Design review of the part built by this model. Coordinates are the model's own, in mm. Face numbers are marked on the shaded views. A direction names the side the tool comes from. Coordinates: 2 decimals unless noted, no trailing zeros. Loops run counter-clockwise (first coordinate to the right, second up) from the corner with the lowest first, then second, coordinate; pieces in that order, holes last. Notation, with made-up numbers: (36, 44) -> (75, 44) arc R11 ccw to (75, 60) -> close; hole circle Ø8 at (-13, -11). An arc over 180 degrees is marked (long way). One line per item, written item: value. Start each with the question number.
1. Add section B-B on z = -12. Write out the cut boundary in (x, y), plus the area to 3 significant figures.
2. Draft analysis for pull direction Z (two halves, no side actions). For the marked faces 4, 5 and 6, state which applies: pulls with the +Z half, pulls with the -Z half, needs draft (parallel to the pull), parting line crosses it, or undercut.
3. Machinability: for the marked faces 1, 2 and 3, which of the approach directions +Z, -Z, +X, -X, +Y, -Y give a long, thin tool a straight path to every point of the face, cutting with its end or side? Answer none if there is none.
4. For probe 1 along X at (y, z) = (11.5, 12); probe 2 along X at (y, z) = (12.75, -6.5); probe 3 along Z at (x, y) = (-4.5, 12), list the stretches that pass through material, from the lowest coordinate up.
5. Insertion check: pin 1 (2 mm diameter, centred on x = 14.5, y = 18.5, fed in from -Z); pin 2 (8 mm diameter, centred on x = 7, z = -13, fed in from +Y); pin 3 (3.5 mm diameter, centred on x = 13.5, z = -9.5, fed in from +Y). Each pin has a flat end and moves straight along its axis. Give the tip position at first contact, or say it passes through.
6. Add section A-A on y = 16. Write out the cut boundary in (x, z).
7. Add section C-C on y = 5.5. Write out the cut boundary in (x, z), plus the area to 3 significant figures.
8. Add section D-D on z = 21. Write out the cut boundary in (x, y).
Autodesk Inventor part; units mm, degrees
ref_plane "YZ Plane" through (0, 0, 0) normal (1, 0, 0) x (0, 1, 0)
ref_plane "XZ Plane" through (0, 0, 0) normal (0, 1, 0) x (-1, 0, 0)
ref_plane "XY Plane" through (0, 0, 0) normal (0, 0, 1) x (1, 0, 0)
sketch "Sketch1" plane through (0, 0, 0) normal (0, 0, 1) x (1, 0, 0)
  line L0 (16.85, 0) -> (-16.85, 0)
  line L1 (-16.85, 0) -> (-16.85, 20)
  line L2 (-16.85, 20) -> (-1.85, 20)
  line L3 (-1.85, 20) -> (-1.85, 7)
  line L4 (-1.85, 7) -> (1.85, 7)
  line L5 (1.85, 7) -> (1.85, 20)
  line L6 (1.85, 20) -> (16.85, 20)
  line L7 (16.85, 20) -> (16.85, 0)
  line L8 (-23.59, 0) -> (23.59, 0)
  line L9 (0, -4) -> (0, 24)
  point P0 (0, 0)
  point P1 (0, 7)
  point P2 (0, 0)
  dimension "d0" = 33.7
  dimension "d1" = 3.7
  dimension "d2" = 13
  dimension "d3" = 20
extrude "Extrusion1" add sketch "Sketch1" along normal mid plane 60
sketch "Sketch2" plane through (-16.85, 20, 30) normal (0, 1, 0) x (1, 0, 0)
  line L0 (0, 60) -> (0, 0)
  line L1 (15, 0) -> (0, 0)
  line L2 (15, 60) -> (15, 0)
  line L3 (0, 60) -> (15, 60)
  line L4 (18.7, 60) -> (18.7, 0)
  line L5 (33.7, 0) -> (18.7, 0)
  line L6 (33.7, 60) -> (33.7, 0)
  line L7 (18.7, 60) -> (33.7, 60)
  line L8 (25.85, 42) -> (7.85, 42) construction
  line L9 (7.85, 42) -> (7.85, 18) construction
  line L10 (7.85, 18) -> (25.85, 18) construction
  line L11 (25.85, 18) -> (25.85, 42) construction
  line L12 (25.85, 42) -> (7.85, 18) construction
  line L13 (7.85, 42) -> (25.85, 18) construction
  point P0 (16.85, 30)
  dimension "d6" = 18
  dimension "d7" = 24
hole "Hole1" at (-9, 20, 12) at (-9, 20, -12) at (9, 20, 12) at (9, 20, -12) direction (0, -1, 0) diameter 4.5 end through all counterbore diameter 12 counterbore depth 3
sketch "Sketch3" plane through (1.85, 20, 30) normal (0, 1, 0) x (1, 0, 0)
  circle A0 centre (-10.85, 18) radius 6
  circle A1 centre (-10.85, 42) radius 6
  line L0 (-18.7, 60) -> (-18.7, 0)
  line L1 (-3.7, 0) -> (-18.7, 0)
  line L2 (-3.7, 60) -> (-3.7, 0)
  line L3 (-18.7, 60) -> (-3.7, 60)
  circle A2 centre (7.15, 18) radius 6
  circle A3 centre (7.15, 42) radius 6
  line L4 (0, 60) -> (0, 0)
  line L5 (15, 0) -> (0, 0)
  line L6 (15, 60) -> (15, 0)
  line L7 (0, 60) -> (15, 60)
  line L8 (7.15, 12) -> (15, 12)
  line L9 (15, 12) -> (15, 24)
  line L10 (15, 24) -> (7.15, 24)
  line L11 (7.15, 24) -> (7.15, 12)
  line L12 (7.15, 36) -> (15, 36)
  line L13 (15, 36) -> (15, 48)
  line L14 (15, 48) -> (7.15, 48)
  line L15 (7.15, 48) -> (7.15, 36)
  line L16 (-18.7, 36) -> (-10.85, 36)
  line L17 (-10.85, 36) -> (-10.85, 48)
  line L18 (-10.85, 48) -> (-18.7, 48)
  line L19 (-18.7, 48) -> (-18.7, 36)
  line L20 (-18.7, 12) -> (-10.85, 12)
  line L21 (-10.85, 12) -> (-10.85, 24)
  line L22 (-10.85, 24) -> (-18.7, 24)
  line L23 (-18.7, 24) -> (-18.7, 12)
  circle A4 centre (7.15, 18) radius 6
  circle A5 centre (7.15, 42) radius 6
  point P0 (-1.85, 30)
extrude "Extrusion2" cut sketch "Sketch3" against normal blind 3 contours L21 A0 | A0 L20 L0 L22 | L0 L18 A1 L16 | A1 L17 | A2 L11 | A2 L10 L6 L8 | L12 A3 L14 L6 | L15 A3 picked at (-12.72, 18.7092) picked at (-12.72, 42.7092) picked at (8.397, 19.5637) picked at (8.7137, 43.247)
fillet "Fillet1" radius 4 4 edges at (-16.85, 10, 30) (16.85, 10, 30) (16.85, 10, -30) (-16.85, 10, -30)
chamfer "Chamfer1" distance 1 angle 45 12 edges at (3, 20, -12) (12.925, 20, -18) (12.925, 20, -6) (-12.925, 20, -18) (-3, 20, -12) (-12.925, 20, -6) (-12.925, 20, 6) (-3, 20, 12) (-12.925, 20, 18) (3, 20, 12) (12.925, 20, 6) (12.925, 20, 18)
chamfer "Chamfer2" distance 1 angle 45 4 edges at (-9, 0, 9.75) (9, 0, 9.75) (-9, 0, -14.25) (9, 0, -14.25)
sketch "Sketch4" plane through (16.85, 17, 18) normal (1, 0, 0) x (0, 0, -1)
  line L0 (-3, -5) -> (39, -5) construction
  line L1 (18, -21) -> (18, 7)
  line L2 (-1, 3) -> (-8, 3)
  point P0 (18, -17)
  point P1 (18, -5)
  dimension "d24" = 42
  dimension "d25" = 8
hole "Hole2" at (16.85, 12, 21) at (16.85, 12, -21) direction (-1, 0, 0) diameter 4 end through all
chamfer "Chamfer3" distance 1 angle 45 4 edges at (16.85, 12, 23) (16.85, 12, -19) (-16.85, 12, -19) (-16.85, 12, 23)
properties part number "sujetador plancha aluminio"
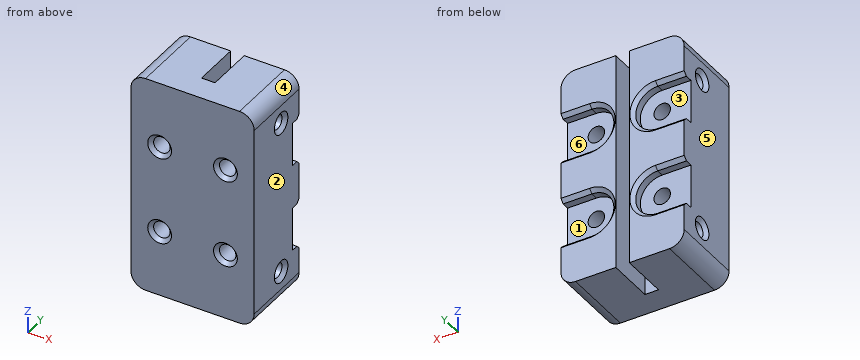
Worked answers:
1. outline: (-16.85, 0) -> (-12.25, 0) -> (-11.25, 1) -> (-11.25, 17) -> (-16.85, 17) -> close; (-6.75, 1) -> (-5.75, 0) -> (5.75, 0) -> (6.75, 1) -> (6.75, 17) -> (3, 17) -> (3, 19) -> (2, 20) -> (1.85, 20) -> (1.85, 7) -> (-1.85, 7) -> (-1.85, 20) -> (-2, 20) -> (-3, 19) -> (-3, 17) -> (-6.75, 17) -> close; (11.25, 1) -> (12.25, 0) -> (16.85, 0) -> (16.85, 17) -> (11.25, 17) -> close
1. area: 387 mm²
2. face 4: pulls with the +Z half
2. face 5: needs draft
2. face 6: undercut
3. face 1: +X, +Y
3. face 2: +Z, -Z, +X, +Y, -Y
3. face 3: -X, +Y
4. probe 1: x = -16.85 to -11.25, -6.75 to -1.85, 1.85 to 6.75, 11.25 to 16.85
4. probe 2: x = -16.85 to -1.85, 1.85 to 16.85
4. probe 3: z = -30 to -23, -19 to 19, 23 to 30
5. pin 1: stops at z = -29.95
5. pin 2: stops at y = 19.24
5. pin 3: stops at y = 17
6. outline: (-16.85, -26) arc R4 ccw to (-12.85, -30) -> (-1.85, -30) -> (-1.85, 30) -> (-12.85, 30) arc R4 ccw to (-16.85, 26) -> close; (1.85, -30) -> (12.85, -30) arc R4 ccw to (16.85, -26) -> (16.85, 26) arc R4 ccw to (12.85, 30) -> (1.85, 30) -> close; hole circle Ø4.5 at (-9, -12); hole circle Ø4.5 at (-9, 12); hole circle Ø4.5 at (9, -12); hole circle Ø4.5 at (9, 12)
7. outline: (-16.85, -26) arc R4 ccw to (-12.85, -30) -> (12.85, -30) arc R4 ccw to (16.85, -26) -> (16.85, 26) arc R4 ccw to (12.85, 30) -> (-12.85, 30) arc R4 ccw to (-16.85, 26) -> close; hole circle Ø4.5 at (-9, -12); hole circle Ø4.5 at (-9, 12); hole circle Ø4.5 at (9, -12); hole circle Ø4.5 at (9, 12)
7. area: 1,940 mm²
8. outline: (-16.85, 0) -> (16.85, 0) -> (16.85, 9) -> (15.85, 10) -> (1.85, 10) -> (1.85, 7) -> (-1.85, 7) -> (-1.85, 10) -> (-15.85, 10) -> (-16.85, 9) -> close; (-16.85, 15) -> (-15.85, 14) -> (-1.85, 14) -> (-1.85, 20) -> (-16.85, 20) -> close; (1.85, 14) -> (15.85, 14) -> (16.85, 15) -> (16.85, 20) -> (1.85, 20) -> close
